Source: CAD feature listing. Evaluate the final solid. Frame: model axes, mm. Face numbers are marked on the shaded views. A direction names the side the tool comes from. Round coordinates to 2 decimals unless told otherwise and drop trailing zeros. Loops run counter-clockwise (first coordinate to the right, second up) from the corner with the lowest first, then second, coordinate; pieces in that order, holes last.
(1) Section C-C, the plane x = -3. Return the cut outline in (y, z).
(2) Mould query, pull axis Y, two halves, no side actions, for the marked faces 3, 4, 5 and 6. Classes: pulls with the +Y half, pulls with the -Y half, needs draft (parallel to the pull), parting line crosses it, or undercut.
(3) Section B-B, the plane z = -1.8. Return the cut outline in (x, y), plus the area to 3 significant figures.
(4) First-contact query: pin 1 Ø3 at (y, z) = (4.5, -2.5) entering from -X; pin 2 Ø1.5 at (x, y) = (-4.5, 6) entering from +Z; pin 3 Ø1.5 at (y, z) = (6, -3) entering from -X. Flat tips, straight axial feed; report the tip coordinate or a pass-through.
(5) Set-up query: the marked faces 1 and 2. Return all of +Z, -Z, +X, -X, +Y, -Y with unobstructed straight access to the full face (end or side cutting, diameter ignored); none if empty.
(6) Material intervals for probe 1 along Y at (x, z) = (-3, -4.9); probe 2 along Y at (x, z) = (-0.45, -3); probe 3 along Z at (x, y) = (-2.85, 6), sorted ascending.
(7) Section A-A, the plane y = 3.5. Return the cut outline in (x, z).
(8) Section D-D, the plane y = 1.5. Return the cut outline in (x, z), plus the area to 3 significant figures.
Autodesk Inventor part; units mm, degrees
ref_plane "YZ Plane" through (0, 0, 0) normal (1, 0, 0) x (0, 1, 0)
ref_plane "XZ Plane" through (0, 0, 0) normal (0, 1, 0) x (-1, 0, 0)
ref_plane "XY Plane" through (0, 0, 0) normal (0, 0, 1) x (1, 0, 0)
sketch "Sketch1" plane through (0, 0, 0) normal (0, 1, 0) x (-1, 0, 0)
  line L0 (0, 0) -> (0, -6)
  line L1 (0, -6) -> (6, -6)
  line L2 (6, -6) -> (0, 0)
  dimension "d0" = 6
  dimension "d1" = 6
extrude "Extrusion1" add sketch "Sketch1" along normal blind 7
ref_plane "Work Plane1" through (-6, 0, 0) normal (1, 0, 0) x (0, 0, -1)
fillet "Fillet1" radius 0.5 1 edges at (0, 3.5, -6)
sketch "Sketch2" plane through (-6, 0, 0) normal (1, 0, 0) x (0, 0, -1)
  line L0 (0, 0) -> (0, 7)
  line L1 (0, 6.25) -> (5, 6.25)
  line L2 (5, 6.25) -> (5, 0.75)
  line L3 (5, 0.75) -> (0, 0.75)
  line L4 (0, 0.75) -> (0, 6.25)
  line L5 (6, 7) -> (0, 7)
  point P0 (0, 0.75)
  dimension "d6" = 5.5
  dimension "d7" = 5
  dimension "d8" = 0.75
extrude "Extrusion2" cut sketch "Sketch2" along normal blind 5
sketch "Sketch3" plane through (-1, 0, 0) normal (-1, 0, 0) x (0, 0, 1)
  circle A0 centre (-3, 3.5) radius 1.5
  line L0 (-6, 0) -> (0, 0)
  dimension "d11" = 3
  dimension "d12" = 3.5
  dimension "d13" = 3
extrude "Extrusion3" cut sketch "Sketch3" against normal blind 5
sketch "Sketch4" plane through (-5, 0.75, -5) normal (0, 0, 1) x (1, 0, 0)
  circle A0 centre (2, 2.75) radius 1.5
  line L0 (-1, 7.65) -> (-1, -2.15)
  line L1 (-1, -0.75) -> (5, -0.75)
  dimension "d16" = 3
  dimension "d17" = 3
  dimension "d18" = 3.5
extrude "Extrusion4" cut sketch "Sketch4" against normal blind 5
fillet "Fillet2" radius 0.5 1 edges at (-6, 3.5, -6)
fillet "Fillet3" radius 0.5 1 edges at (0, 3.5, 0)
properties part number "bracket"
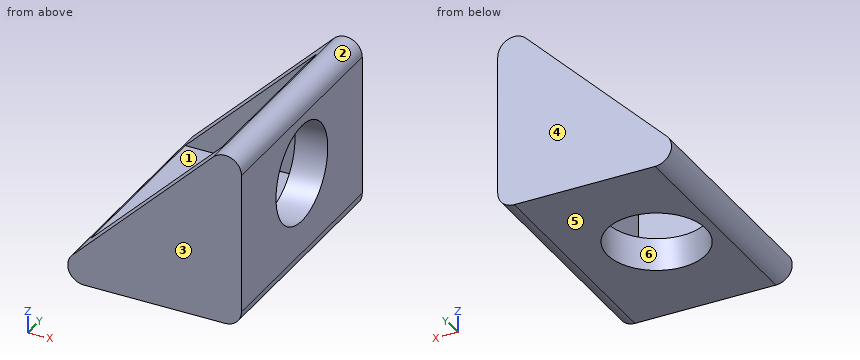
Output values:
1. outline: (0, -6) - (2, -6) - (2, -5) - (0.75, -5) - (0.75, -3) - (0, -3) - close; (5, -6) - (7, -6) - (7, -3) - (6.25, -3) - (6.25, -5) - (5, -5) - close
2. face 3: pulls with the -Y half
2. face 4: pulls with the +Y half
2. face 5: needs draft
2. face 6: undercut
3. outline: (-1.8, 0) - (0, 0) - (0, 2.6) - (-1, 2.6) - (-1, 0.75) - (-1.8, 0.75) - close; (-1.8, 6.25) - (-1, 6.25) - (-1, 4.4) - (0, 4.4) - (0, 7) - (-1.8, 7) - close
3. area: 6.40 mm2
4. pin 1: stops at x = -1
4. pin 2: stops at z = -3.79
4. pin 3: stops at x = -3.71
5. face 1: +Z, -X
5. face 2: +Z, +Y, -Y
6. probe 1: y = 0 to 0.75, 6.25 to 7
6. probe 2: y = 0 to 2, 5 to 7
6. probe 3: z = -6 to -5
7. outline: (-5.15, -5.15) arc R0.5 ccw to (-4.79, -6) - (-4.5, -6) - (-4.5, -5) - (-5, -5) - close; (-1.5, -6) - (-0.5, -6) arc R0.5 ccw to (0, -5.5) - (0, -4.5) - (-1, -4.5) - (-1, -5) - (-1.5, -5) - close; (-1, -1.5) - (0, -1.5) - (0, -1.21) arc R0.5 ccw to (-0.85, -0.85) - (-1, -1) - close
8. outline: (-5.15, -5.15) arc R0.5 ccw to (-4.79, -6) - (-0.5, -6) arc R0.5 ccw to (0, -5.5) - (0, -1.21) arc R0.5 ccw to (-0.85, -0.85) - (-1, -1) - (-1, -5) - (-5, -5) - close
8. area: 9.33 mm2
